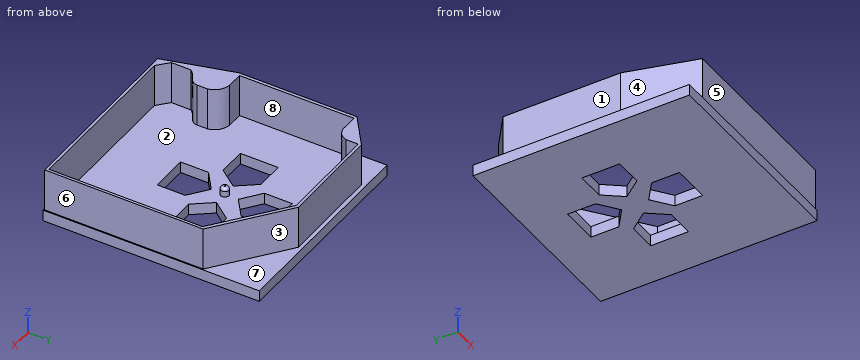
from build123d import *

# Parameters (mm, degrees)
F0_W     = 460
F0_H     = 480
F1_DEPTH = 25
F3_DEPTH = 120
F5_DEPTH = 25
F4_R     = 9
F6_DEPTH = 45
F7_R     = 7


with BuildPart() as f1:
    # F0 (on Top) → F1 (new body)
    with BuildSketch(Plane.XY):
        with Locations((-7.875566, -26.590223)):
            Rectangle(F0_W, F0_H)
    extrude(amount=F1_DEPTH)

    # F2 (on Top) → F3 (join)
    with BuildSketch(Plane.XY):
        Polygon((67.823559, 204.918116), (-160.820395, 204.088688), (-230.491832, 151.282176), (-230.491832, -109.70924), (-187.456321, -264.258176), (219.884232, -264.258176), (219.884232, 87.416694), align=None)
        with BuildLine():
            Line((-159.161553, 170.635357), (-159.161553, 198.282734))
            Line((-159.161553, 198.282734), (65.256598, 198.282734))
            Line((65.256598, 198.282734), (214.078277, 82.440153))
            Line((214.078277, 82.440153), (214.078277, -258.175731))
            Line((214.078277, -258.175731), (-166.073412, -258.175731))
            Line((-166.073412, -258.175731), (-190.403104, -235.951498))
            Line((-190.403104, -235.951498), (-190.403104, -192.651421))
            add(Edge.make_bspline(
                [(-156.396821, -157.539219), (-156.12036, -176.339447), (-179.620609, -176.062971), (-190.403104, -192.651421)],
                knots=[0, 0, 0, 0, 48.880405, 48.880405, 48.880405, 48.880405], degree=3))
            Line((-156.396821, -157.539219), (-156.396821, -134.315416))
            add(Edge.make_bspline(
                [(-156.396821, -134.315416), (-159.714505, -120.768197), (-167.455778, -109.156288), (-187.638372, -105.009183)],
                knots=[0, 0, 0, 0, 42.835614, 42.835614, 42.835614, 42.835614], degree=3))
            Line((-187.638372, -105.009183), (-223.579988, -105.009183))
            Line((-223.579988, -105.009183), (-223.579988, 148.793906))
            Line((-223.579988, 148.793906), (-184.873641, 148.793906))
            add(Edge.make_bspline(
                [(-184.873641, 148.793906), (-169.114619, 152.388066), (-165.243983, 156.81164), (-159.161553, 170.635357)],
                knots=[0, 0, 0, 0, 33.736634, 33.736634, 33.736634, 33.736634], degree=3))
        make_face(mode=Mode.SUBTRACT)
    extrude(amount=F3_DEPTH)

    # F4 (on Top) → F5 (cut, through all)
    with BuildSketch(Plane.XY):
        Polygon((0, 124), (-42, 124), (-42, 62), (0, 30), (42, 62), (42, 124), align=None)
        Polygon((124, 0), (124, 42), (62, 42), (30, 0), (62, -42), (124, -42), align=None)
        Polygon((-124, 0), (-124, -42), (-62, -42), (-30, 0), (-62, 42), (-124, 42), align=None)
        Polygon((0, -124), (42, -124), (42, -62), (0, -30), (-42, -62), (-42, -124), align=None)
    extrude(amount=F5_DEPTH, mode=Mode.SUBTRACT)

    # F4 (on Top) → F6 (join)
    with BuildSketch(Plane.XY):
        Circle(F4_R)
    extrude(amount=F6_DEPTH)

    # F7
    f7_edges = [f1.edges().sort_by_distance(p)[0] for p in [
        (-9, 0, 45),
    ]]
    fillet(f7_edges, radius=F7_R)


solid = f1.part
Design review of the part built by this model. Coordinates are the model's own, in mm. Face numbers are marked on the shaded views. A direction names the side the tool comes from. Round coordinates to 2 decimals unless told otherwise and drop trailing zeros. Loops run counter-clockwise (first coordinate to the right, second up) from the corner with the lowest first, then second, coordinate; pieces in that order, holes last. Notation, with made-up numbers: (35.25, 71) - (72.25, 71) arc R23 ccw to (72.25, 79) - close; hole circle Ø8 at (38, 7.25). An arc over 180 degrees is marked (long way). One line per question, with ' | ' between items.
1. Draft analysis for pull direction X (two halves, no side actions). For the marked faces 6, 7 and 8, state which applies: released by +X, released by -X, zero draft, split by the parting line, or undercut.
Results are:
face 6: released by +X | face 7: zero draft | face 8: undercut
2. We need section C-C, the plane x = 54. State the section outline as (y, z) points.
Results are:
outline: (-266.59, 0) - (-31.5, 0) - (-31.5, 25) - (-258.18, 25) - (-258.18, 120) - (-264.26, 120) - (-264.26, 25) - (-266.59, 25) - close; (31.5, 0) - (213.41, 0) - (213.41, 25) - (204.87, 25) - (204.87, 120) - (198.28, 120) - (198.28, 25) - (31.5, 25) - close
3. We need section A-A, the plane y = 72.5. State the section outline as (x, z) points, and give its area (3 significant figures).
Results are:
outline: (-237.88, 0) - (-42, 0) - (-42, 25) - (-223.58, 25) - (-223.58, 120) - (-230.49, 120) - (-230.49, 25) - (-237.88, 25) - close; (42, 0) - (222.12, 0) - (222.12, 25) - (219.88, 25) - (219.88, 120) - (214.08, 120) - (214.08, 25) - (42, 25) - close | area: 10,600 mm²
4. For the marked faces 1, 2, 3, 4 and 5, list the 3-axis set-ups (+Z, -Z, +X, -X, +Y, -Y) from which the entire face can be reached by the end or side of a thin tool; tool diameter is ignored.
Results are:
face 1: +Z, -X, +Y, -Y | face 2: +Z | face 3: +Z, +X, +Y | face 4: +Z, -X, -Y | face 5: +Z, +X, -X, -Y
5. For L1, parallel to X at y = -3, z = 50; L2, parallel to Y at x = 56.5, z = 80; L3, parallel to X at y = -100, z = 24.5, list the stretches that pass through material, from the lowest coordinate up. Write a range as [from, to].
Results are:
L1: x = [-230.49, -223.58], [214.08, 219.88] | L2: y = [-264.26, -258.18], [198.28, 204.88] | L3: x = [-237.88, -42], [42, 222.12]
6. Clearance check with flat-ended pins moving along their axes: P1, Ø3, axis at x = -58.5, y = -193, coming from the +Z side; P2, Ø4, axis at y = -169.5, z = 91, coming from the +X side; P3, Ø8, axis at x = 122, z = 36, coming from the +Y side. State where each tip first meets the part, or that it passes through.
Results are:
P1: stops at z = 25 | P2: stops at x = 219.88 | P3: stops at y = 166.15
7. We need section B-B, the plane z = 12.5. State the section outline as (x, y) points.
Results are:
outline: (-237.88, -266.59) - (222.12, -266.59) - (222.12, 213.41) - (-237.88, 213.41) - close; hole (-124, -42) - (-62, -42) - (-30, 0) - (-62, 42) - (-124, 42) - close; hole (-42, -124) - (42, -124) - (42, -62) - (0, -30) - (-42, -62) - close; hole (-42, 62) - (0, 30) - (42, 62) - (42, 124) - (-42, 124) - close; hole (30, 0) - (62, -42) - (124, -42) - (124, 42) - (62, 42) - close
